Work out the finished part from the listing and answer in its coordinate system (mm). Give positions to 0.01 mm unless a question says otherwise; leave off trailing zeros. Loops run counter-clockwise (first coordinate to the right, second up) from the corner with the lowest first, then second, coordinate; pieces in that order, holes last.
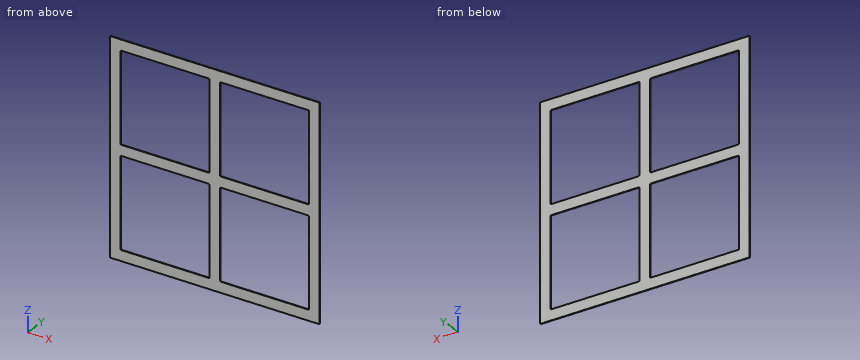
from build123d import *

# Parameters (mm, degrees)
F1_DEPTH = 3


with BuildPart() as f1:
    # F0 (on Front) → F1 (new body)
    with BuildSketch(Plane.XZ):
        with BuildLine():
            ThreePointArc((500, 495), (498.535534, 498.535534), (495, 500))
            Line((495, 500), (-495, 500))
            ThreePointArc((-495, 500), (-498.535534, 498.535534), (-500, 495))
            Line((-500, 495), (-500, -495))
            ThreePointArc((-500, -495), (-498.535534, -498.535534), (-495, -500))
            Line((-495, -500), (495, -500))
            ThreePointArc((495, -500), (498.535534, -498.535534), (500, -495))
            Line((500, -495), (500, 495))
        make_face()
        with BuildLine():
            ThreePointArc((-445, -450), (-448.535534, -448.535534), (-450, -445))
            Line((-450, -445), (-450, -30))
            ThreePointArc((-450, -30), (-448.535534, -26.464466), (-445, -25))
            Line((-445, -25), (-30, -25))
            ThreePointArc((-30, -25), (-26.464466, -26.464466), (-25, -30))
            Line((-25, -30), (-25, -445))
            ThreePointArc((-25, -445), (-26.464466, -448.535534), (-30, -450))
            Line((-30, -450), (-445, -450))
        make_face(mode=Mode.SUBTRACT)
        with BuildLine():
            ThreePointArc((30, -450), (26.464466, -448.535534), (25, -445))
            Line((25, -445), (25, -30))
            ThreePointArc((25, -30), (26.464466, -26.464466), (30, -25))
            Line((30, -25), (445, -25))
            ThreePointArc((445, -25), (448.535534, -26.464466), (450, -30))
            Line((450, -30), (450, -445))
            ThreePointArc((450, -445), (448.535534, -448.535534), (445, -450))
            Line((445, -450), (30, -450))
        make_face(mode=Mode.SUBTRACT)
        with BuildLine():
            ThreePointArc((-25, 30), (-26.464466, 26.464466), (-30, 25))
            Line((-30, 25), (-445, 25))
            ThreePointArc((-445, 25), (-448.535534, 26.464466), (-450, 30))
            Line((-450, 30), (-450, 445))
            ThreePointArc((-450, 445), (-448.535534, 448.535534), (-445, 450))
            Line((-445, 450), (-30, 450))
            ThreePointArc((-30, 450), (-26.464466, 448.535534), (-25, 445))
            Line((-25, 445), (-25, 30))
        make_face(mode=Mode.SUBTRACT)
        with BuildLine():
            ThreePointArc((30, 25), (26.464466, 26.464466), (25, 30))
            Line((25, 30), (25, 445))
            ThreePointArc((25, 445), (26.464466, 448.535534), (30, 450))
            Line((30, 450), (445, 450))
            ThreePointArc((445, 450), (448.535534, 448.535534), (450, 445))
            Line((450, 445), (450, 30))
            ThreePointArc((450, 30), (448.535534, 26.464466), (445, 25))
            Line((445, 25), (30, 25))
        make_face(mode=Mode.SUBTRACT)
    extrude(amount=F1_DEPTH)


solid = f1.part
Item 1: Find section C-C, the plane y = -1.9. Give the number of separate pieces and of enclosed holes in the cut face, plus the area to 3 significant figures.
Item 2: Find section A-A, the plane x = 166. Write down the section's boundary in (y, z), plus the area to 3 significant figures.
Item 3: Find section B-B, the plane z = -147.5. Write down the section's boundary in (x, y), plus the area to 3 significant figures.
Item 4: Consider line 1 (Z direction, x = 197, y = -0.4). Determine where the line is inside the solid, lowest interval first.
Ans:
1. separate pieces: 1
1. enclosed holes: 4
1. area: 278,000 mm2
2. outline: (-3, -500) - (0, -500) - (0, -450) - (-3, -450) - close; (-3, -25) - (0, -25) - (0, 25) - (-3, 25) - close; (-3, 450) - (0, 450) - (0, 500) - (-3, 500) - close
2. area: 450 mm2
3. outline: (-500, -3) - (-450, -3) - (-450, 0) - (-500, 0) - close; (-25, -3) - (25, -3) - (25, 0) - (-25, 0) - close; (450, -3) - (500, -3) - (500, 0) - (450, 0) - close
3. area: 450 mm2
4. line 1: z = -500 to -450, -25 to 25, 450 to 500
